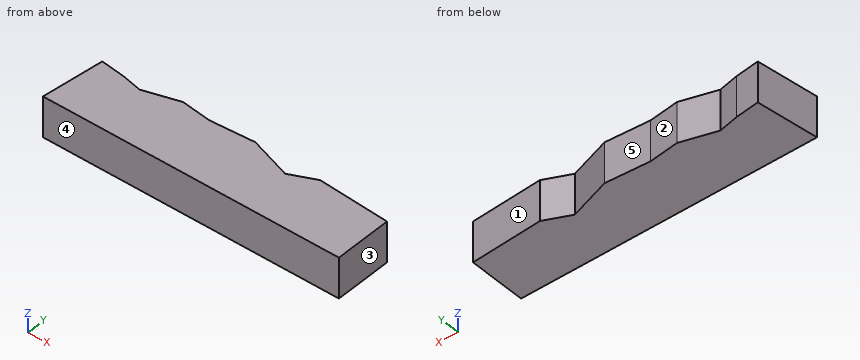
from build123d import *

# Parameters (mm, degrees)
BOSS_EXTRUDE1_DEPTH = 25


with BuildPart() as part:
    # Sketch1 → Boss-Extrude1 (new, symmetric)
    with BuildSketch(Plane.XY):
        Polygon((174.222136922, -57.238128372), (87.15683818, -51.742312172), (56.135286368, -65.87093973), (5.042318242, -48.839950355), (-48.693389614, -52.363603329), (-84.909116911, -47.973818202), (-127.676365392, -60.518877757), (-152.347514605, -55.299980807), (-181.277343289, -51.793334906), (-190.375943184, -126.856784041), (174.222136922, -126.856784041), align=None)
    extrude(amount=BOSS_EXTRUDE1_DEPTH, both=True)


solid = part.part
Here's how the part is built. I have some questions about the finished solid (model axes, mm). Face numbers are marked on the shaded views. A direction names the side the tool comes from. Round coordinates to 2 decimals unless told otherwise and drop trailing zeros. Loops run counter-clockwise (first coordinate to the right, second up) from the corner with the lowest first, then second, coordinate; pieces in that order, holes last.
1. If we section it at B-B on y = -73.5: Write out the boundary of the cut face in (x, z), plus the area to 3 significant figures.
Answer list:
outline: (-183.91, -25) - (174.22, -25) - (174.22, 25) - (-183.91, 25) - close
area: 17,900 mm2
2. If we section it at A-A on z = -3: Write out the boundary of the cut face in (x, y).
Answer list:
outline: (-190.38, -126.86) - (174.22, -126.86) - (174.22, -57.24) - (87.16, -51.74) - (56.14, -65.87) - (5.04, -48.84) - (-48.69, -52.36) - (-84.91, -47.97) - (-127.68, -60.52) - (-152.35, -55.3) - (-181.28, -51.79) - close
3. If we section it at C-C on x = -89: Write out the boundary of the cut face in (y, z).
Answer list:
outline: (-126.86, -25) - (-49.17, -25) - (-49.17, 25) - (-126.86, 25) - close
4. Which directions (+Z, -Z, +X, -X, +Y, -Y) give clear straight access to the entire face, cutting with the end or side of a thin tool? Please do the marked faces 1 and 2.
Answer list:
face 1: +Z, -Z, +X, +Y
face 2: +Z, -Z, +Y
5. For P1, Ø10, axis at y = -69, z = -20, coming from the -X side; P2, Ø6, axis at y = -89, z = -0.5, coming from the -X side; P3, Ø12, axis at x = -114.5, z = -6, coming from the +Y side, each with a flat end and sliding along its axis, tell me the tip position at first contact or that it passes through.
Answer list:
P1: stops at x = -183.97
P2: stops at x = -186.15
P3: stops at y = -54.89
6. If I drill on line 1 along X through (y, z) = (-115, -3.5); line 2 along X through (y, z) = (-93, -1.5); line 3 along Y through (x, z) = (-62, 11), over which ranges is the centre line in solid material (lowest first)?
Answer list:
line 1: x = -188.94 to 174.22
line 2: x = -186.27 to 174.22
line 3: y = -126.86 to -50.75
7. We'd pull the mould along X, two halves only. Please class the marked faces 3, 4 and 5: +X half, -X half, draft (parallel to the pull), parting line (faces both ways), or undercut.
Answer list:
face 3: +X half
face 4: draft
face 5: undercut
